The listing builds one solid part. Answer for the finished solid, in the listing's coordinates (mm). Face numbers are marked on the shaded views. A direction names the side the tool comes from. Give positions to 0.01 mm unless a question says otherwise; leave off trailing zeros. Order: outer loops, then holes, each group sorted by start corner. A loop starts at its lowest first (then second) coordinate and runs counter-clockwise, first axis right, second up.
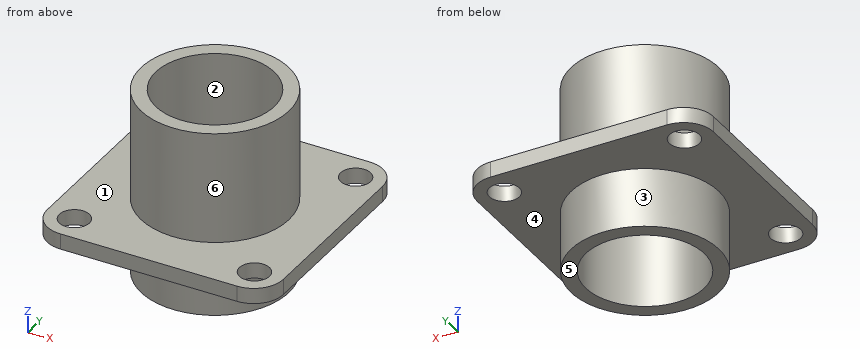
```python
from build123d import *

# Parameters (mm, degrees)
SKETCH_1_W                  = 23.93
SKETCH_1_H                  = 23.93
EXTRUDE_1_DEPTH             = 1.58
SKETCH_2_W                  = 7.495
SKETCH_2_H                  = 11.3
SKETCH_3_W                  = 7.49
SKETCH_3_H                  = 7.44
HOLE_WIZARD_M2_51_D         = 3.05
HOLE_WIZARD_M2_51_DEPTH     = 12.88
HOLE_WIZARD_12_0_12_1_D     = 12
HOLE_WIZARD_12_0_12_1_DEPTH = 10
FILLET_1_R                  = 3
CUT_EXTRUDE_START           = -15
SKETCH_8_R                  = 6
CUT_EXTRUDE_1_DEPTH         = 15
SKETCH_9_R                  = 7.49
SKETCH_9_R_2                = 6
CUT_EXTRUDE_3_DEPTH         = 1.44


with BuildPart() as part:
    # Эскиз1 → Бобышка-Вытянуть1 (new body)
    with BuildSketch(Plane(origin=(0, 0, 0), x_dir=(-1, 0, 0), z_dir=(0, 0, -1))):
        Rectangle(SKETCH_1_W, SKETCH_1_H)
    extrude(amount=-EXTRUDE_1_DEPTH)

    # Эскиз2 → Повернуть1 (revolve)
    with BuildSketch(Plane(origin=(0, 0, 0), x_dir=(1, 0, 0), z_dir=(0, 1, 0))):
        with Locations((3.7475, -7.23)):
            Rectangle(SKETCH_2_W, SKETCH_2_H)
    revolve(axis=Axis((0, 0, 1.58), (0, 0, 1)))

    # Эскиз3 → Повернуть2 (revolve)
    with BuildSketch(Plane.XZ, mode=Mode.PRIVATE) as revolve_2_sk:
        with Locations((3.745, -3.72)):
            Rectangle(SKETCH_3_W, SKETCH_3_H)
    revolve(revolve_2_sk.sketch.rotate(Axis((0, 0, 0), (0, 0, -1)), 180), axis=Axis((0, 0, 0), (0, 0, -1)))

    # Отверстие с зазором M2.51
    with Locations(Plane(origin=(0, 0, 0), x_dir=(-1, 0, 0), z_dir=(0, 0, -1))):
        with Locations((9.13, -9.13), (9.13, 9.13), (-9.13, 9.13), (-9.13, -9.13)):
            Hole(HOLE_WIZARD_M2_51_D / 2, depth=HOLE_WIZARD_M2_51_DEPTH)

    # Диаметр отверстия Ø12.0 (12)1
    with Locations(Plane.XY.offset(12.88)):
        with Locations((0, 0)):
            Hole(HOLE_WIZARD_12_0_12_1_D / 2, depth=HOLE_WIZARD_12_0_12_1_DEPTH)

    # Скругление1
    fillet_1_edges = [part.edges().sort_by_distance(p)[0] for p in [
        (11.965, -11.965, 0.79),
        (11.965, 11.965, 0.79),
        (-11.965, 11.965, 0.79),
        (-11.965, -11.965, 0.79),
    ]]
    fillet(fillet_1_edges, radius=FILLET_1_R)

    # Эскиз8 → Вырез-Вытянуть1 (cut)
    with BuildSketch(Plane.XY.offset(2.88).offset(CUT_EXTRUDE_START)):
        Circle(SKETCH_8_R)
    extrude(amount=CUT_EXTRUDE_1_DEPTH, mode=Mode.SUBTRACT)

    # Эскиз9 → Вырез-Вытянуть3 (cut)
    with BuildSketch(Plane(origin=(0, 0, -7.44), x_dir=(-1, 0, 0), z_dir=(0, 0, -1))):
        Circle(SKETCH_9_R)
        with Locations(Location((0, 0, 0), (0, 0, 180))):
            Circle(SKETCH_9_R_2, mode=Mode.SUBTRACT)
    extrude(amount=-CUT_EXTRUDE_3_DEPTH, mode=Mode.SUBTRACT)


solid = part.part
```
1) Find section C-C (z = 1.25). Write down the section's boundary in (x, y) (3 decimals), then the cut area to 3 significant figures.
Geometry says:
outline: (-11.965, -8.965) arc R3 ccw to (-8.965, -11.965) - (8.965, -11.965) arc R3 ccw to (11.965, -8.965) - (11.965, 8.965) arc R3 ccw to (8.965, 11.965) - (-8.965, 11.965) arc R3 ccw to (-11.965, 8.965) - close; hole circle Ø3.05 at (-9.13, -9.13); hole circle Ø3.05 at (-9.13, 9.13); hole circle Ø12 at (0, 0); hole circle Ø3.05 at (9.13, -9.13); hole circle Ø3.05 at (9.13, 9.13)
area: 423 mm2
2) Straight lines are drawn through the part: probe 1 along Y at (x, z) = (9.13, 0.4) (3 decimals); probe 2 along Y at (x, z) = (0, -0.5); probe 3 along Z at (x, y) = (-6.75, -5.25). For each, find the intervals that lie inside material, in ascending order.
Geometry says:
probe 1: y = -11.96 to -10.655, -7.605 to 7.605, 10.655 to 11.96
probe 2: y = -7.49 to -6, 6 to 7.49
probe 3: z = 0 to 1.58
3) A tool of negligible diameter and unlimited length cuts with its end or side. For the marked faces 4, 5 and 6, from which of +Z, -Z, +X, -X, +Y, -Y can it reach the whole face along a straight path? Write none if from no direction.
Geometry says:
face 4: -Z
face 5: -Z, +X, -X, +Y, -Y
face 6: +Z
4) For a pull along Y with two mould halves and no side action, classify the marked faces 1, 2 and 3 as +Y half, -Y half, draft (parallel to the pull), parting line (faces both ways), or undercut.
Geometry says:
face 1: draft
face 2: undercut
face 3: parting line
5) Given P1, Ø1.5, axis at x = -6.5, z = -3, coming from the +Y side; P2, Ø7, axis at x = 3.5, y = 2, coming from the -Z side; P3, Ø4, axis at x = -9.13, y = 9.13, coming from the -Z side; P4, Ø6, axis at y = 8.5, z = 8, coming from the +X side, each flat-ended and moving along its own axis, determine where each tip first touches the part or whether it passes through.
Geometry says:
P1: stops at y = 4.8
P2: stops at z = -6
P3: stops at z = 0
P4: stops at x = 5.09
6) Find section A-A (x = 0). Write down the section's boundary in (y, z) (3 decimals).
Geometry says:
outline: (-11.965, 0) - (-7.49, 0) - (-7.49, -6) - (-6, -6) - (-6, 12.88) - (-7.495, 12.88) - (-7.495, 1.58) - (-11.965, 1.58) - close; (6, -6) - (7.49, -6) - (7.49, 0) - (11.965, 0) - (11.965, 1.58) - (7.495, 1.58) - (7.495, 12.88) - (6, 12.88) - close
7) Find section D-D (x = -8). Write down the section's boundary in (y, z) (3 decimals).
Geometry says:
outline: (-11.965, 0) - (-10.154, 0) - (-10.154, 1.58) - (-11.965, 1.58) - close; (-8.106, 0) - (8.106, 0) - (8.106, 1.58) - (-8.106, 1.58) - close; (10.154, 0) - (11.965, 0) - (11.965, 1.58) - (10.154, 1.58) - close
